```python
from build123d import *

# Parameters (mm, degrees)
SKETCH1_W           = 20
SKETCH1_H           = 3.8
BOSS_EXTRUDE1_DEPTH = 4.45
SKETCH2_W           = 0.5
SKETCH2_H           = 8.9
BOSS_EXTRUDE2_DEPTH = 1.4
LPATTERN1_COUNT     = 7
LPATTERN1_PITCH     = 2.1
SKETCH3_R           = 2.5
CUT_EXTRUDE1_DEPTH  = 21.838486029


with BuildPart() as part:
    # Sketch1 → Boss-Extrude1 (new, symmetric)
    with BuildSketch(Plane.XY):
        with Locations((-10, 1.9)):
            Rectangle(SKETCH1_W, SKETCH1_H)
    extrude(amount=BOSS_EXTRUDE1_DEPTH, both=True)

    # Sketch2 → Boss-Extrude2 (add)
    with BuildSketch(Plane(origin=(0, 3.8, 0), x_dir=(1, 0, 0), z_dir=(0, 1, 0))):
        with Locations((-19.75, 0)):
            Rectangle(SKETCH2_W, SKETCH2_H)
    boss_extrude2 = extrude(amount=BOSS_EXTRUDE2_DEPTH)

    # LPattern1: Boss-Extrude2 ×7
    with Locations(*[(i * LPATTERN1_PITCH, 0, 0) for i in range(1, LPATTERN1_COUNT)]):
        add(boss_extrude2)

    # Mirror1: part across plane


with BuildPart() as part_1:
    add(part.part)
    add(part.part.mirror(Plane(origin=(0, 0, 4.45), x_dir=(0, 0, 1), z_dir=(-1, 0, 0))))

    # Sketch3 → Cut-Extrude1 (cut, through all)
    with BuildSketch(Plane(origin=(0, 3.8, 0), x_dir=(1, 0, 0), z_dir=(0, 1, 0))):
        with Locations(Location((0, 0, 0), (0, 0, 180))):
            Circle(SKETCH3_R)
    extrude(amount=-CUT_EXTRUDE1_DEPTH, mode=Mode.SUBTRACT)


solid = part_1.part
```
Geometry check sheet. Reference: the model listing, model coordinates, mm. A direction names the side the tool comes from. Coordinates: 2 decimals unless noted, no trailing zeros. Loops run counter-clockwise (first coordinate to the right, second up) from the corner with the lowest first, then second, coordinate; pieces in that order, holes last.
Item 1: Thickness scan on line 1 (Z direction, x = 0, y = 2.8); line 2 (Y direction, x = 17, z = 0.75); line 3 (Z direction, x = 0.5, y = 1.55). Record the ranges inside material, lowest first.
Item 2: Sectioned sample at B-B, the plane y = 0.55. Record the boundary of the cut face in (x, z), then the cut area to 3 significant figures.
Item 3: Release check for a two-part mould opening along X. For faces 3 (the face through (-17.9, 4, 0)), 4 (the face through (0, 2, -4.45)), 5 (the face through (-17.4, 4, 0)) record: released by +X, released by -X, zero draft, split by the parting line, or undercut.
Item 4: Sectioned sample at A-A, the plane x = 0. Record the boundary of the cut face in (y, z), then the cut area to 3 significant figures.
Item 5: Go/stop test with a flat-tipped pin: pin 1 Ø1.3 at (x, z) = (14.5, -1.5) entering from +Y. Record where the tip stops, or that it passes through.
Item 6: Access from +Z, -Z, +X, -X, +Y, -Y to the whole of each face (thin tool, end or side, straight path). Record for faces 1 (the face through (-15.3, 4, 0)), 2 (the face through (2.5, 1.9, 0.1)).
Item 7: Sectioned sample at C-C, the plane x = 8.5. Record the boundary of the cut face in (y, z), then the cut area to 3 significant figures.
Check result:
1. line 1: z = -4.45 to -2.5, 2.5 to 4.45
1. line 2: y = 0 to 3.8
1. line 3: z = -4.45 to -2.45, 2.45 to 4.45
2. outline: (-20, -4.45) - (20, -4.45) - (20, 4.45) - (-20, 4.45) - close; hole circle Ø5 at (0, 0)
2. area: 336 mm2
3. face 3: undercut
3. face 4: zero draft
3. face 5: undercut
4. outline: (0, -4.45) - (3.8, -4.45) - (3.8, -2.5) - (0, -2.5) - close; (0, 2.5) - (3.8, 2.5) - (3.8, 4.45) - (0, 4.45) - close
4. area: 14.8 mm2
5. pin 1: stops at y = 3.8
6. face 1: +Z, -Z, +Y
6. face 2: +Y, -Y
7. outline: (0, -4.45) - (3.8, -4.45) - (3.8, 4.45) - (0, 4.45) - close
7. area: 33.8 mm2
